```python
from build123d import *

# Parameters (mm, degrees)
SKETCH1_W                     = 200
SKETCH1_H                     = 70
BOSS_EXTRUDE1_DEPTH           = 40
SHAFTFITS_REACH               = 115.248
SKETCH2_R                     = 2.75
SKETCH3_R                     = 8.075
PULLEY_DEPTH                  = 30
SKETCH4_R                     = 30
GEARS_FITS_DEPTH              = 10
GEAR_LETOUT_REACH             = 115.248
SKETCH5_W                     = 200
SKETCH5_H                     = 13
CLOSED_LOOP_TIMING_BELT_REACH = 115.248
SKETCH8_W                     = 120
SKETCH8_H                     = 3
SKETCH6_R                     = 32
GEAR_MARGIN_DEPTH             = 10
SKETCH7_R                     = 10.075
PULLEY_MARGIN_DEPTH           = 20


with BuildPart() as part:
    # Sketch1 → Boss-Extrude1 (new body)
    with BuildSketch(Plane.XY):
        Rectangle(SKETCH1_W, SKETCH1_H)
    extrude(amount=BOSS_EXTRUDE1_DEPTH)

    # Sketch2 → ShaftFits (cut, up to next)
    with BuildSketch(Plane.XY.offset(40), mode=Mode.PRIVATE) as shaftfits_sk1:
        with Locations((60, 0)):
            Circle(SKETCH2_R)
    shaftfits_tool1 = extrude(shaftfits_sk1.sketch, amount=-SHAFTFITS_REACH, mode=Mode.PRIVATE) & part.part
    # Sketch2 → ShaftFits (cut, up to next)
    with BuildSketch(Plane.XY.offset(40), mode=Mode.PRIVATE) as shaftfits_sk2:
        with Locations(Location((-60, 0, 0), (0, 0, 180))):
            Circle(SKETCH2_R)
    shaftfits_tool2 = extrude(shaftfits_sk2.sketch, amount=-SHAFTFITS_REACH, mode=Mode.PRIVATE) & part.part
    add(shaftfits_tool1.solids().sort_by_distance((60, 0, 40))[0], mode=Mode.SUBTRACT)
    add(shaftfits_tool2.solids().sort_by_distance((-60, 0, 40))[0], mode=Mode.SUBTRACT)

    # Sketch3 → Pulley (cut)
    with BuildSketch(Plane.XY.offset(40)):
        with Locations((60, 0)):
            Circle(SKETCH3_R)
        with Locations(Location((-60, 0, 0), (0, 0, 180))):
            Circle(SKETCH3_R)
    extrude(amount=-PULLEY_DEPTH, mode=Mode.SUBTRACT)

    # Sketch4 → Gears fits (cut)
    with BuildSketch(Plane.XY.offset(40)):
        with Locations((60, 0)):
            Circle(SKETCH4_R)
        with Locations(Location((-60, 0, 0), (0, 0, 180))):
            Circle(SKETCH4_R)
    extrude(amount=-GEARS_FITS_DEPTH, mode=Mode.SUBTRACT)

    # Sketch5 → Gear letout (cut, up to next)
    with BuildSketch(Plane.XY.offset(40), mode=Mode.PRIVATE) as gear_letout_sk1:
        with Locations((0, -28.5)):
            Rectangle(SKETCH5_W, SKETCH5_H)
    gear_letout_tool1 = extrude(gear_letout_sk1.sketch, amount=-GEAR_LETOUT_REACH, mode=Mode.PRIVATE) & part.part
    add(gear_letout_tool1.solids().sort_by_distance((0, -28.5, 40))[0], mode=Mode.SUBTRACT)

    # Closed-loop timing belt: up to this face of the body (flat: up to its plane)
    closed_loop_timing_belt_end = Plane(part.part.faces().sort_by_distance((-52.15339549, 0, 10))[0])
    # Sketch8 → Closed-loop timing belt (cut, up to the picked face)
    with BuildSketch(Plane.XY.offset(40), mode=Mode.PRIVATE) as closed_loop_timing_belt_sk1:
        with Locations((0, 6.575)):
            Rectangle(SKETCH8_W, SKETCH8_H)
    closed_loop_timing_belt_tool1 = split(extrude(closed_loop_timing_belt_sk1.sketch, amount=-CLOSED_LOOP_TIMING_BELT_REACH, mode=Mode.PRIVATE), bisect_by=closed_loop_timing_belt_end, keep=Keep.BOTH, mode=Mode.PRIVATE)
    # Sketch8 → Closed-loop timing belt (cut, up to the picked face)
    with BuildSketch(Plane.XY.offset(40), mode=Mode.PRIVATE) as closed_loop_timing_belt_sk2:
        with Locations((0, -6.575)):
            Rectangle(SKETCH8_W, SKETCH8_H)
    closed_loop_timing_belt_tool2 = split(extrude(closed_loop_timing_belt_sk2.sketch, amount=-CLOSED_LOOP_TIMING_BELT_REACH, mode=Mode.PRIVATE), bisect_by=closed_loop_timing_belt_end, keep=Keep.BOTH, mode=Mode.PRIVATE)
    add(closed_loop_timing_belt_tool1.solids().sort_by(Axis((0, 6.575, 40), (0, 0, -1)))[0], mode=Mode.SUBTRACT)
    add(closed_loop_timing_belt_tool2.solids().sort_by(Axis((0, -6.575, 40), (0, 0, -1)))[0], mode=Mode.SUBTRACT)

    # Sketch6 → Gear margin (cut)
    with BuildSketch(Plane.XY.offset(40)):
        with Locations((60, 0)):
            Circle(SKETCH6_R)
        with Locations((-60, 0)):
            Circle(SKETCH6_R)
    extrude(amount=-GEAR_MARGIN_DEPTH, mode=Mode.SUBTRACT)

    # Sketch7 → Pulley margin (cut)
    with BuildSketch(Plane.XY.offset(30)):
        with Locations((60, 0)):
            Circle(SKETCH7_R)
        with Locations((-60, 0)):
            Circle(SKETCH7_R)
    extrude(amount=-PULLEY_MARGIN_DEPTH, mode=Mode.SUBTRACT)


solid = part.part
```
Input: part model. Units: mm. Frame: model coordinates. A direction names the side the tool comes from. Coordinates: 2 decimals unless noted, no trailing zeros. Write each loop counter-clockwise with the first axis right and the second up, starting at its lowest first coordinate (ties: lowest second). Pieces come first, ordered by that corner, then holes. Notation, with made-up numbers: M -12,39.5 L 39,39.5 A31 cw 39,63.5 Z; hole C 60,36 d6. An arc over 180 degrees is marked long. Use one line per item in the form item = value.
Q1. Draft query along X for faces 3 (the face through (100, 6, 20)), 4 (the face through (-1, 35, 20)), 5 (the face through (57.253, 0.121, 5.07)). Return one class per face: released by +X, released by -X, zero draft, split by the parting line, or undercut.
Answer below:
face_3 = released by +X
face_4 = zero draft
face_5 = undercut
Q2. Material intervals for probe 1 along Y at (x, z) = (-8.5, 27) (3 decimals); probe 2 along X at (y, z) = (0, 16) (3 decimals); probe 3 along X at (y, z) = (0, 38), sorted ascending. Write a range as from..to.
Answer below:
probe_1 = -22..-8.075, -5.075..5.075, 8.075..35
probe_2 = -100..-70.075, -49.925..49.925, 70.075..100
probe_3 = -100..-92, -28..28, 92..100
Q3. Section B-B (y = 0). Return loops of the section in (x, z) (3 decimals), plus the area to 3 significant figures.
Answer below:
outline = M -100,0 L -62.75,0 L -62.75,10 L -70.075,10 L -70.075,30 L -92,30 L -92,40 L -100,40 Z; M -57.25,0 L 57.25,0 L 57.25,10 L 49.925,10 L 49.925,30 L 28,30 L 28,40 L -28,40 L -28,30 L -49.925,30 L -49.925,10 L -57.25,10 Z; M 62.75,0 L 100,0 L 100,40 L 92,40 L 92,30 L 70.075,30 L 70.075,10 L 62.75,10 Z
area = 5,800 mm²
Q4. Set-up query: faces 1 (the face through (-1, -22, 20)), 2 (the face through (70.07, -0.31, 20.14)). Return all of +Z, -Z, +X, -X, +Y, -Y with unobstructed straight access to the full face (end or side cutting, diameter ignored); none if empty.
Answer below:
face_1 = +Z, -Z, +X, -X, -Y
face_2 = +Z
Q5. First-contact query: pin 1 (7 mm diameter, centred on x = 60, y = 0, fed in from +Z); pin 2 (3 mm diameter, centred on x = 53, y = 13.5, fed in from +Z). Flat tips, straight axial feed; report the tip coordinate or a pass-through.
Answer below:
pin_1 = 10
pin_2 = 30
Q6. Section C-C (z = 32). Return loops of the section in (x, y) (3 decimals), plus the area to 3 significant figures.
Answer below:
outline = M -100,-22 L -83.238,-22 A32 cw long -29.036,8.075 L 29.036,8.075 A32 cw long 83.238,-22 L 100,-22 L 100,35 L -100,35 Z; M -36.762,-22 L 36.762,-22 A32 cw 29.036,-8.075 L -29.036,-8.075 A32 cw Z; M -28.405,-5.075 L 28.405,-5.075 A32 cw 28.405,5.075 L -28.405,5.075 A32 cw Z
area = 5,260 mm²
Q7. Section A-A (x = 60). Return loops of the section in (y, z) (3 decimals), plus the area to 3 significant figures.
Answer below:
outline = M -22,0 L -2.75,0 L -2.75,10 L -10.075,10 L -10.075,30 L -22,30 Z; M 2.75,0 L 35,0 L 35,40 L 32,40 L 32,30 L 10.075,30 L 10.075,10 L 2.75,10 Z
area = 1,280 mm²
Q8. Section D-D (x = -80). Return loops of the section in (y, z).
Answer below:
outline = M -22,0 L 35,0 L 35,40 L 24.98,40 L 24.98,30 L -22,30 Z
